Check sheet for the modelled part. Datum: model origin and axes. Units: mm. Coordinates: 2 decimals unless noted, no trailing zeros. Write each loop counter-clockwise with the first axis right and the second up, starting at its lowest first coordinate (ties: lowest second). Pieces come first, ordered by that corner, then holes. Notation, with made-up numbers: (-6.75, -32) -> (4.25, -32) arc R5 ccw to (4.25, -24) -> close; hole circle Ø3 at (55.25, 54). An arc over 180 degrees is marked (long way). Put each result on its own line as item: value.
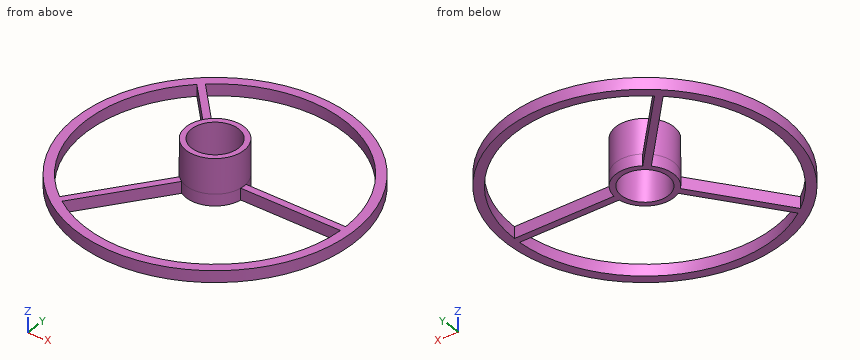
```python
from build123d import *

# Parameters (mm, degrees)
SKETCH_R      = 120
SKETCH_R_2    = 20.3
PAD_DEPTH     = 10
SKETCH001_R   = 25
SKETCH001_R_2 = 20.3
PAD001_DEPTH  = 30


with BuildPart() as part:
    # Sketch → Pad (new body)
    with BuildSketch(Plane.XY):
        Circle(SKETCH_R)
        Circle(SKETCH_R_2, mode=Mode.SUBTRACT)
        with BuildLine():
            ThreePointArc((111.964891, 2.804147), (45.592578, 102.300131), (-72.7719, 85.136658))
            Line((-13.839048, 20.8202), (-72.7719, 85.136658))
            ThreePointArc((24.842237, 2.804147), (10.555192, 22.662478), (-13.839048, 20.8202))
            Line((24.842237, 2.804147), (111.964891, 2.804147))
        make_face(mode=Mode.SUBTRACT)
        with BuildLine():
            Line((24.794913, -3.195666), (111.9544, -3.195666))
            ThreePointArc((-64.872706, -91.299135), (49.94724, -100.246063), (111.9544, -3.195666))
            Line((-13.075988, -21.307711), (-64.872706, -91.299135))
            ThreePointArc((-13.075988, -21.307711), (10.786327, -22.553385), (24.794913, -3.195666))
        make_face(mode=Mode.SUBTRACT)
        with BuildLine():
            Line((-17.776297, -17.578489), (-69.668887, -87.694049))
            ThreePointArc((-77.226732, 81.117395), (-111.88792, -5.009326), (-69.668887, -87.694049))
            Line((-18.401224, 16.923208), (-77.226732, 81.117395))
            ThreePointArc((-18.401224, 16.923208), (-24.9959, -0.452749), (-17.776297, -17.578489))
        make_face(mode=Mode.SUBTRACT)
    extrude(amount=PAD_DEPTH)

    # Sketch001 (on Face16 of Pad) → Pad001 (join)
    with BuildSketch(Plane.XY.offset(10)):
        Circle(SKETCH001_R)
        Circle(SKETCH001_R_2, mode=Mode.SUBTRACT)
    extrude(amount=PAD001_DEPTH)


solid = part.part
```
Q1. Cross-section at C-C (z = 5.5). Record the cut outline in (x, y), plus the area to 3 significant figures.
Recorded:
outline: circle Ø240 at (0, 0); hole (-77.23, 81.12) arc R112 ccw to (-69.67, -87.69) -> (-17.78, -17.58) arc R25 cw to (-18.4, 16.92) -> close; hole (-72.77, 85.14) -> (-13.84, 20.82) arc R25 cw to (24.84, 2.8) -> (111.96, 2.8) arc R112 ccw to start; hole (-64.87, -91.3) arc R112 ccw to (111.95, -3.2) -> (24.79, -3.2) arc R25 cw to (-13.08, -21.31) -> close; hole circle Ø40.6 at (0, 0)
area: 8,070 mm2
Q2. Cross-section at A-A (y = 0). Record the cut outline in (x, z), plus the area to 3 significant figures.
Recorded:
outline: (-120, 0) -> (-112, 0) -> (-112, 10) -> (-120, 10) -> close; (-25, 0) -> (-20.3, 0) -> (-20.3, 40) -> (-25, 40) -> close; (20.3, 0) -> (120, 0) -> (120, 10) -> (25, 10) -> (25, 40) -> (20.3, 40) -> close
area: 1,410 mm2
Q3. Material ranges on line 1 along Y through (x, z) = (1.5, 4); line 2 along Y through (x, z) = (0, 9); line 3 along Y through (x, z) = (0, 11), recorded low to high.
Recorded:
line 1: y = -119.99 to -111.99, -24.95 to -20.24, 20.24 to 24.95, 111.99 to 119.99
line 2: y = -120 to -112, -25 to -20.3, 20.3 to 25, 112 to 120
line 3: y = -25 to -20.3, 20.3 to 25
Q4. Depth check by flat-ended pin: P1, Ø1, axis at x = 86.5, z = 9.5, coming from the +Y side; P2, Ø8, axis at x = 54.5, z = 4, coming from the -Y side; P3, Ø8, axis at x = 88.5, z = 4.5, coming from the +Y side. Enter the tip coordinate at first touch or a pass-through.
Recorded:
P1: stops at y = 83.69
P2: stops at y = -108.86
P3: stops at y = 85.2
Q5. Cross-section at B-B (x = 0). Record the cut outline in (y, z), plus the area to 3 significant figures.
Recorded:
outline: (-120, 0) -> (-112, 0) -> (-112, 10) -> (-120, 10) -> close; (-25, 0) -> (-20.3, 0) -> (-20.3, 40) -> (-25, 40) -> close; (20.3, 0) -> (25, 0) -> (25, 40) -> (20.3, 40) -> close; (112, 0) -> (120, 0) -> (120, 10) -> (112, 10) -> close
area: 536 mm2
Q6. Cross-section at D-D (y = -102). Record the cut outline in (x, z), plus the area to 3 significant figures.
Recorded:
outline: (-63.21, 0) -> (-46.26, 0) -> (-46.26, 10) -> (-63.21, 10) -> close; (46.26, 0) -> (63.21, 0) -> (63.21, 10) -> (46.26, 10) -> close
area: 339 mm2
